CAD build for the part. Positions are in the model's coordinates, mm. Face numbers are marked on the shaded views. A direction names the side the tool comes from. Coordinates: 2 decimals unless noted, no trailing zeros. Write each loop counter-clockwise with the first axis right and the second up, starting at its lowest first coordinate (ties: lowest second). Pieces come first, ordered by that corner, then holes.
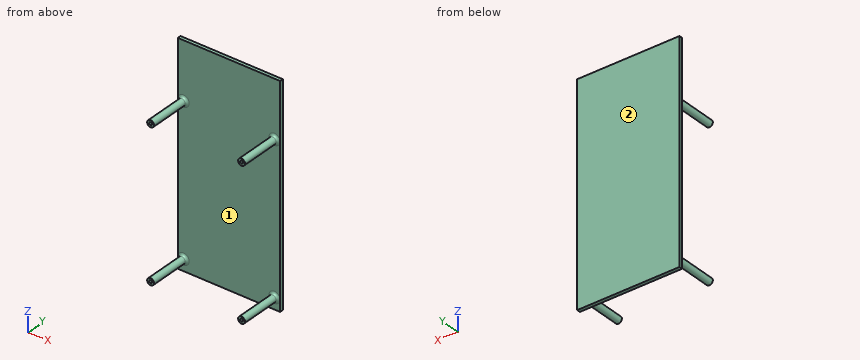
Autodesk Inventor part; units mm, degrees
ref_plane "YZ Plane" through (0, 0, 0) normal (1, 0, 0) x (0, 1, 0)
ref_plane "XZ Plane" through (0, 0, 0) normal (0, 1, 0) x (-1, 0, 0)
ref_plane "XY Plane" through (0, 0, 0) normal (0, 0, 1) x (1, 0, 0)
sketch "Esquisse1" plane through (0, 0, 0) normal (0, 1, 0) x (-1, 0, 0)
  line L0 (0, 0) -> (0, 65)
  line L1 (0, 0) -> (0, -65)
  line L2 (0, 65) -> (40, 65)
  line L3 (-40, -65) -> (40, -65)
  circle A0 centre (40, 65) radius 3
  circle A1 centre (40, -65) radius 3
  circle A2 centre (-40, -65) radius 3
  line L4 (0, 65) -> (-40, 65)
  circle A3 centre (-40, 65) radius 3
  dimension "d0" = 65
  dimension "d1" = 65
  dimension "d2" = 40
  dimension "d4" = 80
  dimension "d5" = 6
  dimension "d7" = 6
  dimension "d9" = 6
  dimension "d11" = 40
  dimension "d12" = 6
extrude "Extrusion1" add sketch "Esquisse1" along normal blind 37
sketch "Esquisse2" plane through (-40, 37, 65) normal (0, 1, 0) x (1, 0, 0)
  line L0 (0, 0) -> (80, 0)
  line L1 (80, 0) -> (80, 130)
  line L2 (80, 130) -> (0, 130)
  line L3 (0, 130) -> (0, 0)
  line L4 (0, 0) -> (0, -10)
  line L5 (0, -10) -> (85, -10)
  line L6 (85, -10) -> (85, 140)
  line L7 (85, 140) -> (-5, 140)
  line L8 (-5, 140) -> (-5, -10)
  line L9 (-5, -10) -> (0, -10)
  point P0 (40, 65)
  dimension "d16" = 80
  dimension "d17" = 130
  dimension "d18" = 10
  dimension "d19" = 85
  dimension "d20" = 150
  dimension "d21" = 90
extrude "Extrusion2" add sketch "Esquisse2" along normal blind 3 contours L3 L2 L1 L0 | L9 L8 L7 L6 L5
sketch "Esquisse3" plane through (40, 0, 65) normal (0, -1, 0) x (1, 0, 0)
  circle A0 centre (0, -130) radius 3
  circle A1 centre (-80, 0) radius 3
  circle A2 centre (-80, -130) radius 3
  point P0 (-40, -65)
  point P1 (0, 0)
hole "Perçage1" at (40, 0, 65) at (40, 0, -65) at (-40, 0, 65) at (-40, 0, -65) direction (0, 1, 0) diameter 2.459 depth 30
sketch "Esquisse4" plane through (-45, 37, 75) normal (0, 0, 1) x (1, 0, 0)
  line L0 (0, 0) -> (90, 0)
  line L1 (90, 0) -> (90, 3)
  line L2 (0, 3) -> (90, 3)
  line L3 (0, 0) -> (0, 3)
  point P0 (45, -37)
extrude "Extrusion3" add sketch "Esquisse4" along normal blind 40
fillet "Congé1" radius 2 4 edges at (-37, 37, 65) (43, 37, 65) (43, 37, -65) (-37, 37, -65)
properties part number "Support intérieur châssis"
Item 1: Saw through at A-A, the plane y = 14. Write the cut outline in (x, z), and give its area (3 significant figures).
Item 2: Saw through at C-C, the plane z = -24. Write the cut outline in (x, y).
Item 3: Which spindle directions (+Z, -Z, +X, -X, +Y, -Y) get a long thin tool onto all of the face, cutting with end or side? Do the marked faces 1 and 2. Say none if no direction does.
Item 4: Saw through at B-B, the plane x = 3.5. Write the cut outline in (y, z).
Item 5: Flat gauge pin, fed straight in: pin 1 Ø1.2 at (x, z) = (-40, 65) entering from -Y. Where does the tip first touch, or does it go through?
Item 6: Wall check: line 1 along Z through (x, y) = (40, 12); line 2 along Y through (x, z) = (-14.5, 95.5). Give the ranges that are in metal, low to high.
Working result:
1. outline: circle Ø6 at (-40, -65); circle Ø6 at (-40, 65); circle Ø6 at (40, -65); circle Ø6 at (40, 65); hole circle Ø2.46 at (-40, -65); hole circle Ø2.46 at (-40, 65); hole circle Ø2.46 at (40, -65); hole circle Ø2.46 at (40, 65)
1. area: 94.1 mm2
2. outline: (-45, 37) - (45, 37) - (45, 40) - (-45, 40) - close
3. face 1: -Y
3. face 2: +Z, -Z, +X, -X, +Y
4. outline: (37, -75) - (40, -75) - (40, 115) - (37, 115) - close
5. pin 1: stops at y = 30
6. line 1: z = -68 to -66.23, -63.77 to -62, 62 to 63.77, 66.23 to 68
6. line 2: y = 37 to 40
